Autodesk Fusion 360 part; units mm, degrees
sketch "Sketch1" plane through (0, 0, 0) normal (0, 0, 1) x (1, 0, 0)
  circle A0 centre (0, 0) radius 45.5
  circle A1 centre (0, 0) radius 46.5
  circle A2 centre (0, 0) radius 44
  dimension "d1" = 91
  dimension "d2" = 93
  dimension "d3" = 88
extrude "Extrude1" add sketch "Sketch1" along normal blind 5 contours A0 | A1 | A2
extrude "Extrude2" add sketch "Sketch1" along normal blind 30 contours A0
extrude "Extrude3" add sketch "Sketch1" along normal blind 35 contours A1
sketch "Sketch2" plane through (0, 0, 5) normal (0, 0, 1) x (-1, 0, 0)
  circle A0 centre (0, 0) radius 44
  line L0 (-24.5, 0) -> (24.5, 0) construction
  line L1 (24.5, 0) -> (24.5, 26) construction
  line L2 (24.5, 26) -> (-24.5, 26) construction
  line L3 (-24.5, 26) -> (-24.5, 0) construction
  circle A1 centre (-24.916, 26.2774) radius 0.5
  circle A2 centre (-25, 0) radius 0.5
  circle A3 centre (24.916, 26.2774) radius 0.5
  circle A4 centre (24.7236, -0.4472) radius 0.5
  dimension "d11" = 49
  dimension "d12" = 26
  dimension "d13" = 1
  dimension "d14" = 1
  dimension "d15" = 1
  dimension "d16" = 1
extrude "Extrude4" add sketch "Sketch2" along normal blind 2 contours A1 | A2 | A3 | A4
sketch "Sketch3" plane through (0, 0, 5) normal (0, 0, 1) x (-1, 0, 0)
  circle A0 centre (-24.916, 26.2774) radius 0.5
  circle A1 centre (24.916, 26.2774) radius 0.5
  circle A2 centre (-25, 0) radius 0.5
  circle A3 centre (24.7236, -0.4472) radius 0.5
  circle A4 centre (0, 0) radius 44
  circle A5 centre (0, -25) radius 7.0711
extrude "Extrude5" cut sketch "Sketch3" against normal blind 6 contours A5
Could you check a few things on this model? Use its own coordinates, in mm. A direction names the side the tool comes from. Round coordinates to 2 decimals unless told otherwise and drop trailing zeros. Write each loop counter-clockwise with the first axis right and the second up, starting at its lowest first coordinate (ties: lowest second). Pieces come first, ordered by that corner, then holes. Notation, with made-up numbers: M 65.5,-14 L 82.5,-14 A19 ccw 82.5,6 Z; hole C 5.5,25.25 d4. An arc over 180 degrees is marked long. Write each question's results on one line, items separated by ' | '. Start each with the question number.
1. Imagine slicing it at B-B on y = -2.5. List the corners of the cut face in (x, z) for me.
2. Imagine slicing it at A-A on x = 0. List the corners of the cut face in (y, z) for me.
3. Imagine slicing it at D-D on y = 25. List the corners of the cut face in (x, z) for me, and give its area (3 significant figures).
4. Thinking about a two-plate mould opening in X: for faces 3 (the face through (44.35, -13.97, 17.26)), 4 (the face through (-1, 1, 0)), 5 (the face through (-36.107, 27.686, 32.465)), which applies, +X half, -X half, draft (parallel to the pull), parting line (faces both ways), or undercut?
5. I'm going to push flat-ended pins straight in: pin 1 Ø1.1 at (x, y) = (25, 0) entering from +Z; pin 2 Ø1 at (x, y) = (10, 12) entering from +Z; pin 3 Ø4 at (y, z) = (28, 14) entering from +X; pin 4 Ø11.5 at (x, y) = (0, 25) entering from +Z (3 decimals). Where does each tip first touch, or does it pass through?
6. On a 3-axis mill with a long thin cutter (end or side, diameter ignored), from which of +Z, -Z, +X, -X, +Y, -Y can I reach the whole of each face in a straight line? I mean faces 1 (the face through (-23.8, 37.3, 30)), 2 (the face through (1, 18, 3)). Say none if no direction works.
7. Imagine slicing it at C-C on z = 25.5. List the corners of the cut face in (x, y) for me, and give its area (3 significant figures).
8. I need wall thicknesses on L1, parallel to Y at x = 0, z = 18.5; L2, parallel to Z at x = 5, y = 4.5; L3, parallel to Y at x = -34.5, z = 13. Which ranges of each line are inside material? Lowest first, please. Write a range as from..to.
Result sheet:
1) outline: M -46.43,0 L 46.43,0 L 46.43,35 L 45.43,35 L 45.43,30 L 43.93,30 L 43.93,5 L -43.93,5 L -43.93,30 L -45.43,30 L -45.43,35 L -46.43,35 Z
2) outline: M -46.5,0 L 17.93,0 L 17.93,5 L -44,5 L -44,30 L -45.5,30 L -45.5,35 L -46.5,35 Z; M 32.07,0 L 46.5,0 L 46.5,35 L 45.5,35 L 45.5,30 L 44,30 L 44,5 L 32.07,5 Z
3) outline: M -39.21,0 L -7.07,0 L -7.07,5 L -36.21,5 L -36.21,30 L -38.02,30 L -38.02,35 L -39.21,35 Z; M 7.07,0 L 39.21,0 L 39.21,35 L 38.02,35 L 38.02,30 L 36.21,30 L 36.21,5 L 7.07,5 Z | area: 483 mm^2
4) face 3: parting line | face 4: draft | face 5: undercut
5) pin 1: stops at z = 7 | pin 2: stops at z = 5 | pin 3: stops at x = 38.55 | pin 4: passes through
6) face 1: +Z | face 2: +Z, -Z
7) outline: C 0,0 d93; hole C 0,0 d88 | area: 711 mm^2
8) L1: y = -46.5..-44, 44..46.5 | L2: z = 0..5 | L3: y = -31.18..-27.31, 27.31..31.18
